CAD build for the part. Positions are in the model's coordinates, mm. Face numbers are marked on the shaded views. A direction names the side the tool comes from. Coordinates: 2 decimals unless noted, no trailing zeros. Order: outer loops, then holes, each group sorted by start corner. A loop starts at its lowest first (then second) coordinate and runs counter-clockwise, first axis right, second up. Notation, with made-up numbers: (34, 33) - (89, 33) arc R15 ccw to (89, 55) - close; hole circle Ø4 at (-29, -26). An arc over 180 degrees is marked (long way). Return JSON: item names as keys, results as strings.
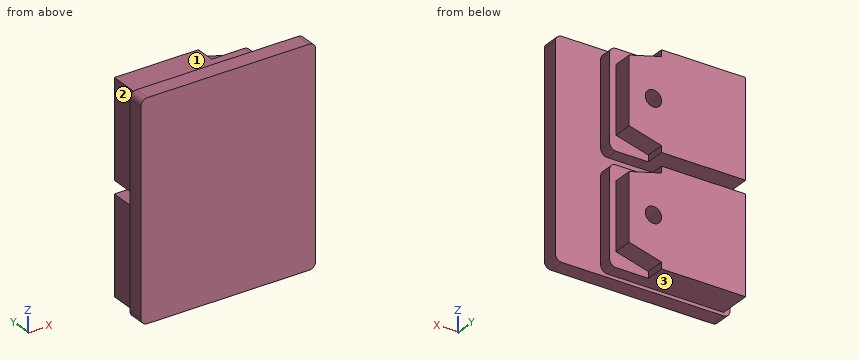
from build123d import *

# Parameters (mm, degrees)
SKETCH1_W              = 27
SKETCH1_H              = 33
EXTRUDE1_DEPTH         = 2.5
FILLET1_R              = 1
SKETCH2_W              = 19
SKETCH2_H              = 15
EXTRUDE2_DEPTH         = 5
CUT_EXTRUDE1_DEPTH     = 3
FILLET2_R              = 1
SKETCH4_R              = 1.25
CUT_EXTRUDE2_DEPTH     = 23.59977876
LPATTERN1_COUNT        = 2
LPATTERN1_PITCH        = 17
FILLET2_OF_LPATTERN1_R = 1
SKETCH5_W              = 8.254105746
SKETCH5_H              = 23.141343318
EXTRUDE3_DEPTH         = 2.5


with BuildPart() as part:
    # Sketch1 → Extrude1 (new body)
    with BuildSketch(Plane(origin=(0, 0, 0), x_dir=(1, 0, 0), z_dir=(0, 1, 0))):
        Rectangle(SKETCH1_W, SKETCH1_H)
    extrude(amount=EXTRUDE1_DEPTH)

    # Fillet1
    fillet1_edges = [part.edges().sort_by_distance(p)[0] for p in [
        (-13.5, 1.25, -16.5),
        (13.5, 1.25, -16.5),
        (13.5, 1.25, 16.5),
        (-13.5, 1.25, 16.5),
    ]]
    fillet(fillet1_edges, radius=FILLET1_R)

    # Sketch2 → Extrude2 (add)
    with BuildSketch(Plane(origin=(0, 2.5, 0), x_dir=(-1, 0, 0), z_dir=(0, 1, 0))):
        with Locations((3, 8.5)):
            Rectangle(SKETCH2_W, SKETCH2_H)
    extrude2 = extrude(amount=EXTRUDE2_DEPTH)

    # Sketch3 → Cut-Extrude1 (cut)
    with BuildSketch(Plane(origin=(0, 7.5, 0), x_dir=(-1, 0, 0), z_dir=(0, 1, 0))):
        Polygon((-0.5, 16), (-6.5, 16), (-6.5, 1), (-0.5, 1), (-0.5, 2), (-5.5, 3.339745962), (-5.5, 13.660254038), (-0.5, 15), align=None)
    cut_extrude1 = extrude(amount=-CUT_EXTRUDE1_DEPTH, mode=Mode.SUBTRACT)

    # Fillet2
    fillet2_edges = [part.edges().sort_by_distance(p)[0] for p in [
        (6.5, 3.5, 1),
        (6.5, 3.5, 16),
    ]]
    fillet(fillet2_edges, radius=FILLET2_R)

    # Sketch4 → Cut-Extrude2 (cut, through all)
    with BuildSketch(Plane(origin=(0, 7.5, 0), x_dir=(-1, 0, 0), z_dir=(0, 1, 0))):
        with Locations(Location((-1.75, 8.5, 0), (0, 0, 90))):
            Circle(SKETCH4_R)
    cut_extrude2 = extrude(amount=-CUT_EXTRUDE2_DEPTH, mode=Mode.SUBTRACT)

    # LPattern1: Extrude2, Cut-Extrude1, Cut-Extrude2 ×2
    with Locations(*[(0, 0, -i * LPATTERN1_PITCH) for i in range(1, LPATTERN1_COUNT)]):
        add(extrude2)
        add(cut_extrude1, mode=Mode.SUBTRACT)
        add(cut_extrude2, mode=Mode.SUBTRACT)

    # Fillet2 of LPattern1
    fillet2_of_lpattern1_edges = [part.edges().sort_by_distance(p)[0] for p in [
        (6.5, 3.5, -16),
        (6.5, 3.5, -1),
    ]]
    fillet(fillet2_of_lpattern1_edges, radius=FILLET2_OF_LPATTERN1_R)

    # Sketch5 → Extrude3 (add)
    with BuildSketch(Plane.XZ):
        with Locations((1.09884186, 0.082461012)):
            Rectangle(SKETCH5_W, SKETCH5_H)
    extrude(amount=-EXTRUDE3_DEPTH)


solid = part.part
Item 1: Band-saw the part on D-D, the plane z = 8.5. List the corners of the cut face in (x, y).
Findings below:
{"outline": "(-13.5, 0) - (13.5, 0) - (13.5, 2.5) - (6.5, 2.5) - (6.5, 4.5) - (5.5, 4.5) - (5.5, 7.5) - (3, 7.5) - (3, 2.5) - (0.5, 2.5) - (0.5, 7.5) - (-12.5, 7.5) - (-12.5, 2.5) - (-13.5, 2.5) - close"}
Item 2: Band-saw the part on C-C, the plane z = 5. List the corners of the cut face in (x, y), then the cut area to 4 significant figures.
Findings below:
{"outline": "(-13.5, 0) - (13.5, 0) - (13.5, 2.5) - (6.5, 2.5) - (6.5, 4.5) - (5.5, 4.5) - (5.5, 7.5) - (-12.5, 7.5) - (-12.5, 2.5) - (-13.5, 2.5) - close", "area": "159.5 mm²"}
Item 3: Band-saw the part on A-A, the plane y = 3.25. List the corners of the cut face in (x, z), then the cut area to 3 significant figures.
Findings below:
{"outline": "(-12.5, -16) - (5.5, -16) arc R1 ccw to (6.5, -15) - (6.5, -2) arc R1 ccw to (5.5, -1) - (-12.5, -1) - close; (-12.5, 1) - (5.5, 1) arc R1 ccw to (6.5, 2) - (6.5, 15) arc R1 ccw to (5.5, 16) - (-12.5, 16) - close; hole circle Ø2.5 at (1.75, -8.5); hole circle Ø2.5 at (1.75, 8.5)", "area": "559 mm²"}
Item 4: Wall check: L1, parallel to Z at x = -3, y = 3.5; L2, parallel to X at y = 3, z = -7.5; L3, parallel to X at y = 6, z = 8.5. Give the ranges that are in metal, low to high. Write a range as [from, to].
Findings below:
{"L1": "z = [-16, -1], [1, 16]", "L2": "x = [-12.5, 1], [2.5, 6.5]", "L3": "x = [-12.5, 0.5], [3, 5.5]"}
Item 5: Which spindle directions (+Z, -Z, +X, -X, +Y, -Y) get a long thin tool onto all of the face, cutting with end or side? Do the marked faces 1, 2 and 3. Say none if no direction does.
Findings below:
{"face 1": "+Z, +X, -X, +Y", "face 2": "+Z, -Z, -X, +Y", "face 3": "-Z, +X, -X, +Y"}
Item 6: Drop flat-ended pins along their axis: P1, Ø4, axis at y = 6, z = -6, coming from the -X side; P2, Ø1.5, axis at x = -3, y = 4, coming from the +Z side; P3, Ø2.5, axis at y = 6, z = 11, coming from the +X side. Give the stop position or say it passes through.
Findings below:
{"P1": "stops at x = -12.5", "P2": "stops at z = 16", "P3": "stops at x = 5.5"}
Item 7: Band-saw the part on B-B, the plane x = -12. List the corners of the cut face in (y, z).
Findings below:
{"outline": "(0, -16.5) - (2.5, -16.5) - (2.5, -16) - (7.5, -16) - (7.5, -1) - (2.5, -1) - (2.5, 1) - (7.5, 1) - (7.5, 16) - (2.5, 16) - (2.5, 16.5) - (0, 16.5) - close"}
